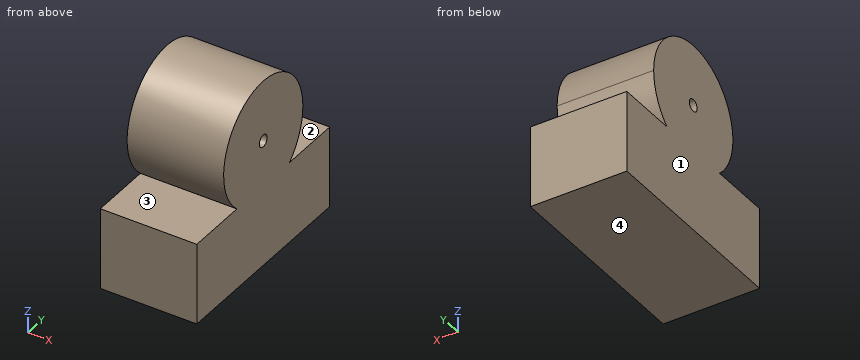
from build123d import *

# Parameters (mm, degrees)
F1_DEPTH = 12.7
F2_DEPTH = 25.4
F4_D     = 6.35


with BuildPart() as f1:
    # F0 (on Right) → F1 (new body, symmetric)
    with BuildSketch(Plane.YZ):
        with BuildLine():
            Line((-54.1098564863, 21.4459784329), (-54.1098564863, -21.4459784329))
            Line((-54.1098564863, -21.4459784329), (54.1098564863, -21.4459784329))
            Line((54.1098564863, -21.4459784329), (54.1098564863, 21.4459784329))
            Line((54.1098564863, 21.4459784329), (21.4569509104, 21.4459784329))
            ThreePointArc((21.4569509104, 21.4459784329), (0, 13.2705383003), (-21.4569509104, 21.4459784329))
            Line((-21.4569509104, 21.4459784329), (-54.1098564863, 21.4459784329))
        make_face()
    extrude(amount=F1_DEPTH, both=True)

    # F0 (on Right) → F2 (join, symmetric)
    with BuildSketch(Plane.YZ):
        with BuildLine():
            Line((-54.1098564863, 21.4459784329), (-54.1098564863, -21.4459784329))
            Line((-54.1098564863, -21.4459784329), (54.1098564863, -21.4459784329))
            Line((54.1098564863, -21.4459784329), (54.1098564863, 21.4459784329))
            Line((54.1098564863, 21.4459784329), (21.4569509104, 21.4459784329))
            ThreePointArc((21.4569509104, 21.4459784329), (0, 13.2705383003), (-21.4569509104, 21.4459784329))
            Line((-21.4569509104, 21.4459784329), (-54.1098564863, 21.4459784329))
        make_face()
        with BuildLine():
            ThreePointArc((32.2452709079, 45.5158092082), (-13.1884855264, 74.9406515262), (-21.4569509104, 21.4459784329))
            Line((-21.4569509104, 21.4459784329), (21.4569509104, 21.4459784329))
            ThreePointArc((21.4569509104, 21.4459784329), (29.4248423181, 32.3273236818), (32.2452709079, 45.5158092082))
        make_face()
        with BuildLine():
            Line((21.4569509104, 21.4459784329), (-21.4569509104, 21.4459784329))
            ThreePointArc((-21.4569509104, 21.4459784329), (0, 13.2705383003), (21.4569509104, 21.4459784329))
        make_face()
    extrude(amount=F2_DEPTH, both=True)

    # F4 (through all)
    with Locations(Plane.YZ.offset(25.4)):
        with Locations((0, 45.5158092082)):
            Hole(F4_D / 2)


solid = f1.part
Geometry check sheet. Reference: the model listing, model coordinates, mm. Face numbers are marked on the shaded views. Give positions to 0.01 mm unless a question says otherwise; leave off trailing zeros. Loops run counter-clockwise (first coordinate to the right, second up) from the corner with the lowest first, then second, coordinate; pieces in that order, holes last.
(1) Section check C-C on y = 44.5. Record the cut outline in (x, z).
From the geometry:
outline: (-25.4, -21.45) - (25.4, -21.45) - (25.4, 21.45) - (-25.4, 21.45) - close
(2) Thickness scan on L1, parallel to Z at x = 11, y = 0; L2, parallel to Z at x = -17, y = -39; L3, parallel to Y at x = 15, z = 44. Record the ranges inside material, lowest first.
From the geometry:
L1: z = -21.45 to 42.34, 48.69 to 77.76
L2: z = -21.45 to 21.45
L3: y = -32.21 to -2.79, 2.79 to 32.21
(3) Depth check by flat-ended pin: pin 1 Ø5 at (y, z) = (0, 45.52) entering from -X; pin 2 Ø3 at (x, z) = (-15, 23.5) entering from -Y; pin 3 Ø2 at (x, y) = (-1, 3.5) entering from +Z; pin 4 Ø10 at (x, y) = (9, -44.5) entering from +Z. Enter the tip coordinate at first touch or a pass-through.
From the geometry:
pin 1: passes through
pin 2: stops at y = -24.88
pin 3: stops at z = 77.66
pin 4: stops at z = 21.45
(4) Release check for a two-part mould opening along Z. For the marked faces 1, 2, 3 and 4 record: released by +Z, released by -Z, zero draft, split by the parting line, or undercut.
From the geometry:
face 1: zero draft
face 2: undercut
face 3: undercut
face 4: released by -Z
(5) Section check B-B on x = -15.5. Record the cut outline in (y, z) (3 decimals), then the cut area to 3 significant figures.
From the geometry:
outline: (-54.11, -21.446) - (54.11, -21.446) - (54.11, 21.446) - (21.457, 21.446) arc R32.245 ccw (long way) to (-21.457, 21.446) - (-54.11, 21.446) - close; hole circle Ø6.35 at (0, 45.516)
area: 7,640 mm2
(6) Section check D-D on y = -23.5. Record the cut outline in (x, z), then the cut area to 3 significant figures.
From the geometry:
outline: (-25.4, -21.45) - (25.4, -21.45) - (25.4, 21.45) - (-25.4, 21.45) - close; (-25.4, 23.44) - (25.4, 23.44) - (25.4, 67.6) - (-25.4, 67.6) - close
area: 4,420 mm2
(7) Section check A-A on y = 0. Record the cut outline in (x, z).
From the geometry:
outline: (-25.4, -21.45) - (25.4, -21.45) - (25.4, 42.34) - (-25.4, 42.34) - close; (-25.4, 48.69) - (25.4, 48.69) - (25.4, 77.76) - (-25.4, 77.76) - close
